Could you check a few things on this model? Use its own coordinates, in mm. A direction names the side the tool comes from. Coordinates: 2 decimals unless noted, no trailing zeros. Loops run counter-clockwise (first coordinate to the right, second up) from the corner with the lowest first, then second, coordinate; pieces in that order, holes last.
1) Imagine slicing it at A-A on y = 0. Please give me the cut outline in (x, z), plus the area to 3 significant figures.
2) Thinking about a two-plate mould opening in X: for faces 4 (the face through (-1.35, 1, 2)), 5 (the face through (1.35, 1, 2)), 6 (the face through (4, 7.35, 2)), 7 (the face through (2.6, 4, 2)), which applies, released by +X, released by -X, zero draft, split by the parting line, or undercut?
3) Imagine slicing it at B-B on z = 5.25. Please give me the cut outline in (x, y), plus the area to 3 significant figures.
4) Will these pins go through, and if not, where does the flat tip stop? P1, Ø2, axis at y = -0.5, z = 1.5, coming from the +X side; P2, Ø1.5, axis at y = 3, z = 2.5, coming from the +X side; P3, Ø0.8, axis at y = 11, z = 2, coming from the -X side.
5) Imagine slicing it at C-C on x = 1.75. Please give me the cut outline in (y, z), plus the area to 4 significant figures.
6) If I drill on line 1 along Y through (x, z) = (2.25, 3.75); line 2 along X through (y, z) = (5.75, 4), over which ranges is the centre line in solid material (lowest first)?
7) For faces 1 (the face through (3, 1.6, 4)), 2 (the face through (3.43, 0.91, 3.08)), 3 (the face through (0, 10.65, 2)), which set-ups out of +Z, -Z, +X, -X, +Y, -Y let a thin tool reach every point of the face, with its end or its side?
```python
from build123d import *

# Parameters (mm, degrees)
PAD017_DEPTH           = 5
PAD020_DEPTH           = 6.25
SKETCH112_W            = 7.5
SKETCH112_H            = 1.65
PAD082_DEPTH           = 5
SKETCH113_W            = 2.1
SKETCH113_H            = 1.65
PAD083_DEPTH           = 5
SKETCH111_W            = 7.5
SKETCH111_H            = 1.65
PAD084_DEPTH           = 5
LINEARPATTERN026_COUNT = 2
LINEARPATTERN026_PITCH = 3.3


with BuildPart() as obj1:
    # Sketch034 → Pad017 (new body)
    with BuildSketch(Plane.XY):
        with BuildLine():
            Line((-1.35, -1.8), (-1.35, 6))
            ThreePointArc((0, 7.35), (-0.954594, 6.954594), (-1.35, 6))
            Line((0, 9), (0, 7.35))
            Line((-2.6, 9), (0, 9))
            Line((-2.6, -1.8), (-2.6, 9))
            Line((-3.85, -1.8), (-2.6, -1.8))
            ThreePointArc((-3.85, -1.8), (-3.439949, -2.789949), (-2.45, -3.2))
            Line((-1.35, -3.2), (-2.45, -3.2))
            Line((-1.35, -1.8), (-1.35, -3.2))
        make_face()
    extrude(amount=PAD017_DEPTH)

    # Sketch037 → Pad020 (join)
    with BuildSketch(Plane.XY):
        Polygon((-1.35, 0.2), (-1.35, 1.6), (-2.6, 1.6), (-3.85, 1.6), (-3, 0.2), (-2.6, 0.2), align=None)
    extrude(amount=PAD020_DEPTH)


with BuildPart() as obj2:
    # Mirror001: instance of _obj1
    add(obj1.part.mirror(Plane(origin=(0, 0, 0), x_dir=(0, 1, 0), z_dir=(-1, 0, 0))))


with BuildPart() as body042:
    # Fusion001 base: copy of _obj1
    add(obj1.part)

    # Fusion001: union _obj2)
    add(obj2.part)

    # Sketch112 → Pad082 (new body)
    with BuildSketch(Plane.XY):
        with Locations((1.15, 8.175)):
            Rectangle(SKETCH112_W, SKETCH112_H)
    pad082 = extrude(amount=PAD082_DEPTH)

    # Sketch113 → Pad083 (join)
    with BuildSketch(Plane.XY):
        with Locations((3.85, 9.825)):
            Rectangle(SKETCH113_W, SKETCH113_H)
    pad083 = extrude(amount=PAD083_DEPTH)

    # Sketch111 → Pad084 (join)
    with BuildSketch(Plane.XY):
        with Locations((1.15, 11.475)):
            Rectangle(SKETCH111_W, SKETCH111_H)
    pad084 = extrude(amount=PAD084_DEPTH)

    # LinearPattern026: Pad083, Pad082, Pad084 ×2
    with Locations(*[(0, i * LINEARPATTERN026_PITCH, 0) for i in range(1, LINEARPATTERN026_COUNT)]):
        add(pad083)
        add(pad082)
        add(pad084)


solid = body042.part
```
Filled in:
1. outline: (-2.6, 0) - (-1.35, 0) - (-1.35, 5) - (-2.6, 5) - close; (1.35, 0) - (2.6, 0) - (2.6, 5) - (1.35, 5) - close
1. area: 12.5 mm2
2. face 4: undercut
2. face 5: undercut
2. face 6: zero draft
2. face 7: released by +X
3. outline: (-3.85, 1.6) - (-3, 0.2) - (-1.35, 0.2) - (-1.35, 1.6) - close; (1.35, 0.2) - (3, 0.2) - (3.85, 1.6) - (1.35, 1.6) - close
3. area: 5.81 mm2
4. P1: stops at x = 3.18
4. P2: stops at x = 2.6
4. P3: stops at x = -2.6
5. outline: (-3.2, 0) - (9, 0) - (9, 5) - (1.6, 5) - (1.6, 6.25) - (0.2, 6.25) - (0.2, 5) - (-3.2, 5) - close; (10.65, 0) - (12.3, 0) - (12.3, 5) - (10.65, 5) - close; (13.95, 0) - (15.6, 0) - (15.6, 5) - (13.95, 5) - close
5. area: 79.25 mm2
6. line 1: y = -3.2 to 9, 10.65 to 12.3, 13.95 to 15.6
6. line 2: x = -2.6 to -1.35, 1.35 to 2.6
7. face 1: +Z, +X
7. face 2: +Z, -Z, +X
7. face 3: +Z, -Z, -X
